Verification items for the finished model (mm, model axes). Face numbers are marked on the shaded views. Coordinates: 2 decimals unless noted, no trailing zeros. Write each loop counter-clockwise with the first axis right and the second up, starting at its lowest first coordinate (ties: lowest second). Pieces come first, ordered by that corner, then holes. Notation, with made-up numbers: (22.25, -0.75) -> (57.25, -0.75) arc R14 ccw to (57.25, 3.25) -> close; hole circle Ø5 at (5, 66.5). An arc over 180 degrees is marked (long way). Use a Markdown table: item, result. Add a question column.
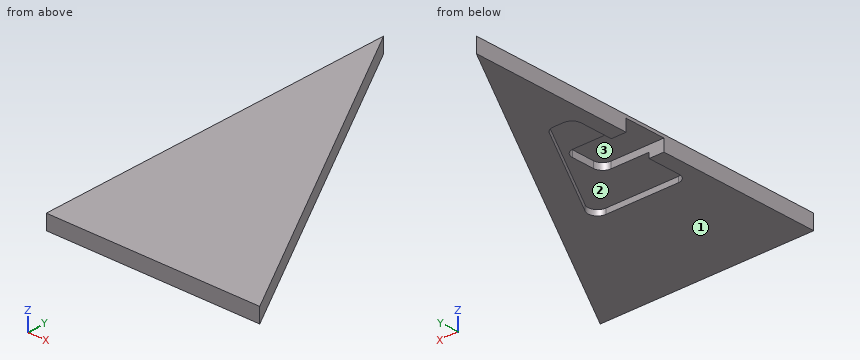
from build123d import *

# Parameters (mm, degrees)
EXTRUDE1_DEPTH = 2.54
EXTRUDE3_DEPTH = 2.032
EXTRUDE2_DEPTH = 0.9144
FILLET1_R      = 1.5875


with BuildPart() as part:
    # Sketch1 → Extrude1 (new body)
    with BuildSketch(Plane.XY):
        Polygon((0, 63.5), (36.6522, 0), (0, 0), align=None)
    extrude(amount=EXTRUDE1_DEPTH)

    # Sketch4 → Extrude3 (cut)
    with BuildSketch(Plane(origin=(0, 0, 0), x_dir=(-1, 0, 0), z_dir=(0, 0, -1))):
        Polygon((0, 31.75), (0, 35.306), (-10.668, 35.306), (-10.668, 28.194), (0, 28.194), align=None)
    extrude(amount=-EXTRUDE3_DEPTH, mode=Mode.SUBTRACT)

    # Sketch3 → Extrude2 (cut)
    with BuildSketch(Plane(origin=(0, 0, 0), x_dir=(-1, 0, 0), z_dir=(0, 0, -1))):
        Polygon((-2.54, 31.75), (-2.54, 20.955), (-19.315938, 20.955), (-6.85419, 42.545), (-2.54, 42.545), align=None)
    extrude(amount=-EXTRUDE2_DEPTH, mode=Mode.SUBTRACT)

    # Fillet1
    fillet1_edges = [part.edges().sort_by_distance(p)[0] for p in [
        (10.668, 28.194, 1.4732),
        (10.668, 35.306, 1.4732),
        (2.54, 42.545, 0.4572),
        (2.54, 20.955, 0.4572),
        (19.315938, 20.955, 0.4572),
        (6.85419, 42.545, 0.4572),
    ]]
    fillet(fillet1_edges, radius=FILLET1_R)


solid = part.part
1) Release check for a two-part mould opening along Y. For the marked faces 1, 2 and 3 record: released by +Y, released by -Y, zero draft, split by the parting line, or undercut.
2) Thickness scan on L1, parallel to Y at x = 13.5, z = 0.3 (3 decimals); L2, parallel to Y at x = 4, z = 0.5; L3, parallel to X at y = 37, z = 1.55. Record the ranges inside material, lowest first.
3) Cross-section at B-B on y = 36. Record the boundary of the cut face in (x, z).
4) Cross-section at A-A on z = 1.35. Record the boundary of the cut face in (x, y) (1 decimal).
5) Gauge pin test, flat ends, axial feed: pin 1 (1 mm diameter, centred on x = 4, z = 0.5, fed in from +Y); pin 2 (1 mm diameter, centred on x = 19.5, y = 22.5, fed in from -Z); pin 3 (0.7 mm diameter, centred on x = 10.5, z = 0.5, fed in from +Y); pin 4 (0.7 mm diameter, centred on y = 39.5, z = 0.5, fed in from +X). Record the tip position at first contact, or that the pin passes through.
6) Cross-section at C-C on x = 26.5. Record the boundary of the cut face in (y, z), then the cut area to 3 significant figures.
7) Cross-section at D-D on y = 10. Record the boundary of the cut face in (x, z), then the cut area to 3 significant figures.
Returned:
| question | item | result |
|---|---|---|
| 1 | face 1 | zero draft |
| 1 | face 2 | undercut |
| 1 | face 3 | undercut |
| 2 | L1 | y = 0 to 20.955, 31.031 to 40.111 |
| 2 | L2 | y = 0 to 20.96, 42.54 to 56.57 |
| 2 | L3 | x = 0 to 15.3 |
| 3 | outline | (0, 0) -> (2.54, 0) -> (2.54, 0.91) -> (10.63, 0.91) -> (10.63, 0) -> (15.87, 0) -> (15.87, 2.54) -> (0, 2.54) -> close |
| 4 | outline | (0, 0) -> (36.7, 0) -> (0, 63.5) -> (0, 35.3) -> (9.1, 35.3) arc R1.6 cw to (10.7, 33.7) -> (10.7, 29.8) arc R1.6 cw to (9.1, 28.2) -> (0, 28.2) -> close |
| 5 | pin 1 | stops at y = 57.44 |
| 5 | pin 2 | stops at z = 0 |
| 5 | pin 3 | stops at y = 45.92 |
| 5 | pin 4 | stops at x = 14.05 |
| 6 | outline | (0, 0) -> (17.59, 0) -> (17.59, 2.54) -> (0, 2.54) -> close |
| 6 | area | 44.7 mm² |
| 7 | outline | (0, 0) -> (30.88, 0) -> (30.88, 2.54) -> (0, 2.54) -> close |
| 7 | area | 78.4 mm² |
